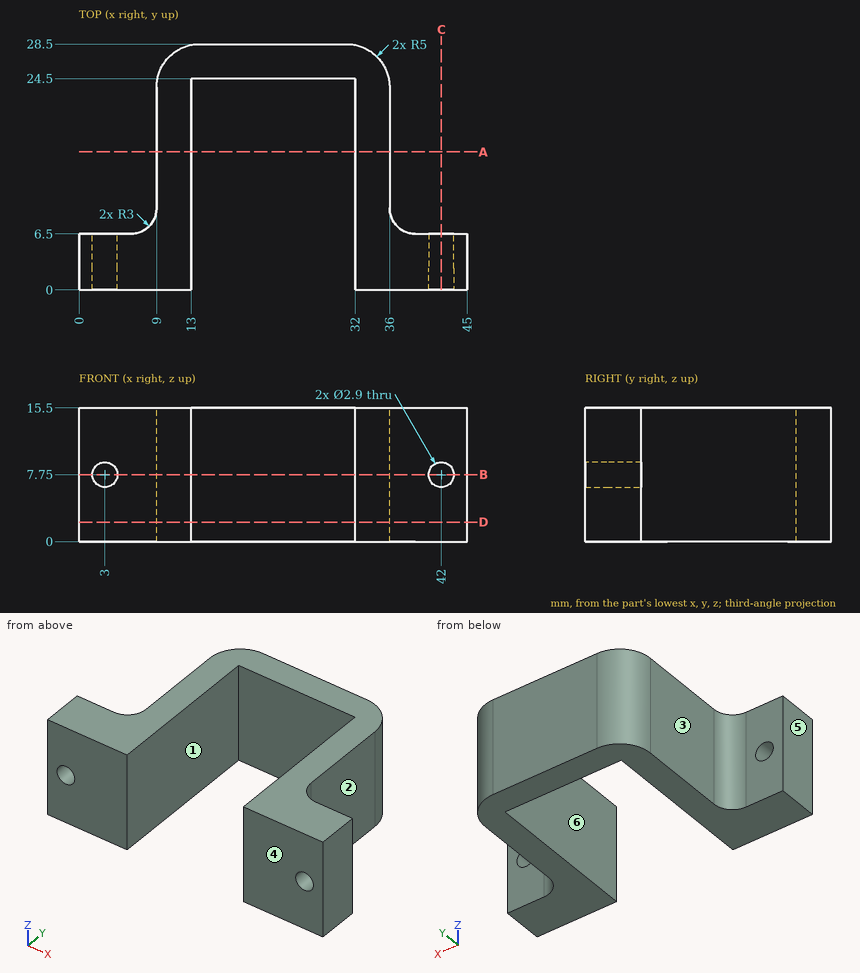
Geometry check sheet. Reference: drawing and pictorial views, mm from the part's lowest x, y, z. A direction names the side the tool comes from. Coordinates: 2 decimals unless noted, no trailing zeros. Write each loop counter-clockwise with the first axis right and the second up, starting at its lowest first coordinate (ties: lowest second). Pieces come first, ordered by that corner, then holes. Notation, with made-up numbers: M 46.25,-12 L 57.25,-12 A16 cw 57.25,3 Z; hole C 7.25,3 d1. An arc over 180 degrees is marked long. Write item = value, one per line. Start each with the question number.
1. Sectioned sample at A-A (y = 16). Record the cut outline in (x, z), then the cut area to 3 significant figures.
2. Tool access check on the marked faces 1, 2 and 3. Record the directions out of +Z, -Z, +X, -X, +Y, -Y that give a thin tool (end or side, any length) a straight path to the whole face; none if there is none.
3. Sectioned sample at C-C (x = 42). Record the cut outline in (y, z), then the cut area to 3 significant figures.
4. Mould release check, pull along X, two halves, no side actions. Record for the marked faces 4, 5 and 6: pulls with the +X half, pulls with the -X half, needs draft (parallel to the pull), parting line crosses it, or undercut.
5. Sectioned sample at B-B (z = 7.75). Record the cut outline in (x, y), then the cut area to 3 significant figures.
6. Go/stop test with flat-tipped pins: pin 1 (12 mm diameter, centred on x = 38.5, y = 14, fed in from +Z); pin 2 (1.8 mm diameter, centred on x = 3, z = 5.5, fed in from +Y); pin 3 (1.5 mm diameter, centred on x = 11.5, z = 10, fed in from +Y); pin 4 (5 mm diameter, centred on y = 18, z = 4, fed in from +X). Record where each tip stops, or that it passes through.
7. Thickness scan on probe 1 along X at (y, z) = (1.25, 7.75); probe 2 along X at (y, z) = (12.25, 4.25); probe 3 along Z at (x, y) = (42, 1.25). Record the ranges inside material, lowest first.
8. Sectioned sample at D-D (z = 2.25). Record the cut outline in (x, y).
The answers:
q1.outline = M 9,0 L 13,0 L 13,15.5 L 9,15.5 Z; M 32,0 L 36,0 L 36,15.5 L 32,15.5 Z
q1.area = 124 mm²
q2.face_1 = +Z, -Z, -Y
q2.face_2 = +Z, -Z, +X, +Y
q2.face_3 = +Z, -Z, -X, +Y
q3.outline = M 0,0 L 6.5,0 L 6.5,6.3 L 0,6.3 Z; M 0,9.2 L 6.5,9.2 L 6.5,15.5 L 0,15.5 Z
q3.area = 81.9 mm²
q4.face_4 = needs draft
q4.face_5 = pulls with the -X half
q4.face_6 = undercut
q5.outline = M 0,0 L 1.55,0 L 1.55,6.5 L 0,6.5 Z; M 4.45,0 L 13,0 L 13,24.5 L 32,24.5 L 32,0 L 40.55,0 L 40.55,6.5 L 39,6.5 A3 cw 36,9.5 L 36,23.5 A5 ccw 31,28.5 L 14,28.5 A5 ccw 9,23.5 L 9,9.5 A3 cw 6,6.5 L 4.45,6.5 Z; M 43.45,0 L 45,0 L 45,6.5 L 43.45,6.5 Z
q5.area = 376 mm²
q6.pin_1 = 15.5
q6.pin_2 = 6.5
q6.pin_3 = 28.18
q6.pin_4 = 36
q7.probe_1 = 0 to 1.55, 4.45 to 13, 32 to 40.55, 43.45 to 45
q7.probe_2 = 9 to 13, 32 to 36
q7.probe_3 = 0 to 6.3, 9.2 to 15.5
q8.outline = M 0,0 L 13,0 L 13,24.5 L 32,24.5 L 32,0 L 45,0 L 45,6.5 L 39,6.5 A3 cw 36,9.5 L 36,23.5 A5 ccw 31,28.5 L 14,28.5 A5 ccw 9,23.5 L 9,9.5 A3 cw 6,6.5 L 0,6.5 Z
